Part print with two shaded views. Sizes in mm from the minimum x, y, z corner. Give positions to 0.01 mm unless a question says otherwise; leave off trailing zeros. Write each loop counter-clockwise with the first axis right and the second up, starting at its lowest first coordinate (ties: lowest second). Pieces come first, ordered by that corner, then holes.
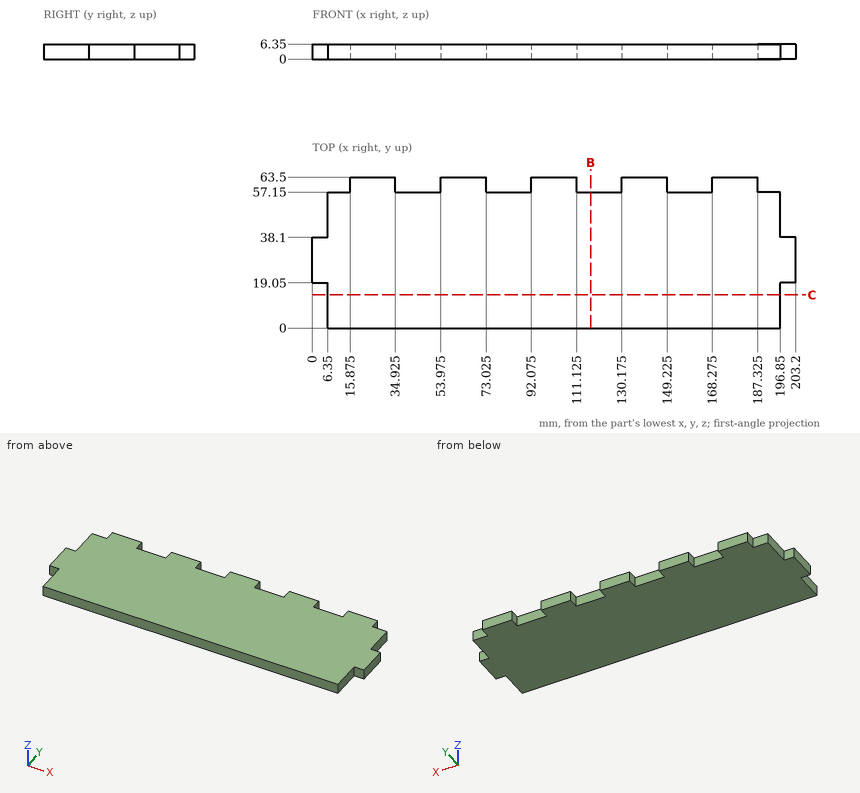
1) Pin check, flat tips, straight feed: pin 1 Ø3 at (x, z) = (80, 4) entering from +Y; pin 2 Ø1.9 at (y, z) = (13, 2) entering from -X; pin 3 Ø3 at (y, z) = (59, 1.5) entering from +X (3 decimals). Stop position of each tip, or through.
Answers follow:
pin 1: stops at y = 57.15
pin 2: stops at x = 6.35
pin 3: stops at x = 187.325
2) Saw through at B-B, the plane x = 117. Write the cut outline in (y, z).
Answers follow:
outline: (0, 0) - (57.15, 0) - (57.15, 6.35) - (0, 6.35) - close
3) Wall check: L1, parallel to X at y = 60.5, z = 2.25 (3 decimals); L2, parallel to X at y = 16, z = 5.25; L3, parallel to Y at x = 117, z = 3.25. Give the ranges that are in metal, low to high.
Answers follow:
L1: x = 15.875 to 34.925, 53.975 to 73.025, 92.075 to 111.125, 130.175 to 149.225, 168.275 to 187.325
L2: x = 6.35 to 196.85
L3: y = 0 to 57.15
4) Saw through at C-C, the plane y = 14. Write the cut outline in (x, z).
Answers follow:
outline: (6.35, 0) - (196.85, 0) - (196.85, 6.35) - (6.35, 6.35) - close
